The listing builds one solid part. Answer for the finished solid, in the listing's coordinates (mm). Face numbers are marked on the shaded views. Coordinates: 2 decimals unless noted, no trailing zeros. Write each loop counter-clockwise with the first axis right and the second up, starting at its lowest first coordinate (ties: lowest second). Pieces come first, ordered by that corner, then holes.
from build123d import *

# Parameters (mm, degrees)
EXTRUDE_1_DEPTH     = 5
SKETCH_4_R          = 1.5
CUT_EXTRUDE_4_DEPTH = 90.180603272
SKETCH_4_3_W        = 111
SKETCH_4_3_H        = 85
SKETCH_4_3_R        = 1.5
CUT_EXTRUDE_5_DEPTH = 3.3
FILLET_1_R          = 2


with BuildPart() as part:
    # Sketch 2 → Extrude 1 (new body)
    with BuildSketch(Plane(origin=(0, 0, 0), x_dir=(1, 0, 0), z_dir=(0, 1, 0))):
        Polygon((-43.3, 45.3), (-43.3, 67.3), (-33.3, 67.3), (-33.3, 45.3), (33.3, 45.3), (33.3, 67.3), (43.3, 67.3), (43.3, 45.3), (58.3, 45.3), (58.3, -45.3), (-58.3, -45.3), (-58.3, 45.3), align=None)
        with BuildLine():
            Line((-35.55, 62.3), (-35.55, 50.3))
            ThreePointArc((-35.55, 50.3), (-38.3, 47.55), (-41.05, 50.3))
            Line((-41.05, 50.3), (-41.05, 62.3))
            ThreePointArc((-41.05, 62.3), (-38.3, 65.05), (-35.55, 62.3))
        make_face(mode=Mode.SUBTRACT)
        with BuildLine():
            Line((35.55, 62.3), (35.55, 50.3))
            ThreePointArc((35.55, 50.3), (38.3, 47.55), (41.05, 50.3))
            Line((41.05, 50.3), (41.05, 62.3))
            ThreePointArc((41.05, 62.3), (38.3, 65.05), (35.55, 62.3))
        make_face(mode=Mode.SUBTRACT)
    extrude(amount=EXTRUDE_1_DEPTH)

    # Sketch 4 → Cut-Extrude 4 (cut, through all)
    with BuildSketch(Plane(origin=(0, 5, 0), x_dir=(1, 0, 0), z_dir=(0, 1, 0))):
        with Locations(Location((-51.5, 38.5, 0), (0, 0, 270))):
            Circle(SKETCH_4_R)
        with Locations(Location((-51.5, -38.5, 0), (0, 0, 270))):
            Circle(SKETCH_4_R)
        with Locations(Location((51.5, -38.5, 0), (0, 0, 270))):
            Circle(SKETCH_4_R)
        with Locations(Location((51.5, 38.5, 0), (0, 0, 270))):
            Circle(SKETCH_4_R)
    extrude(amount=-CUT_EXTRUDE_4_DEPTH, mode=Mode.SUBTRACT)

    # Sketch 4_3 → Cut-Extrude 5 (cut)
    with BuildSketch(Plane(origin=(0, 5, 0), x_dir=(1, 0, 0), z_dir=(0, 1, 0))):
        Rectangle(SKETCH_4_3_W, SKETCH_4_3_H)
        with Locations(Location((-51.5, -38.5, 0), (0, 0, 270))):
            Circle(SKETCH_4_3_R, mode=Mode.SUBTRACT)
        with Locations(Location((-51.5, 38.5, 0), (0, 0, 270))):
            Circle(SKETCH_4_3_R, mode=Mode.SUBTRACT)
        with Locations(Location((51.5, -38.5, 0), (0, 0, 270))):
            Circle(SKETCH_4_3_R, mode=Mode.SUBTRACT)
        with Locations(Location((51.5, 38.5, 0), (0, 0, 270))):
            Circle(SKETCH_4_3_R, mode=Mode.SUBTRACT)
    extrude(amount=-CUT_EXTRUDE_5_DEPTH, mode=Mode.SUBTRACT)

    # Fillet 1
    fillet_1_edges = [part.edges().sort_by_distance(p)[0] for p in [
        (-58.3, 2.5, -45.3),
        (-43.3, 2.5, -45.3),
        (-43.3, 2.5, -67.3),
        (-33.3, 2.5, -67.3),
        (-33.3, 2.5, -45.3),
        (33.3, 2.5, -45.3),
        (33.3, 2.5, -67.3),
        (43.3, 2.5, -67.3),
        (43.3, 2.5, -45.3),
        (58.3, 2.5, -45.3),
        (58.3, 2.5, 45.3),
        (-58.3, 2.5, 45.3),
    ]]
    fillet(fillet_1_edges, radius=FILLET_1_R)


solid = part.part
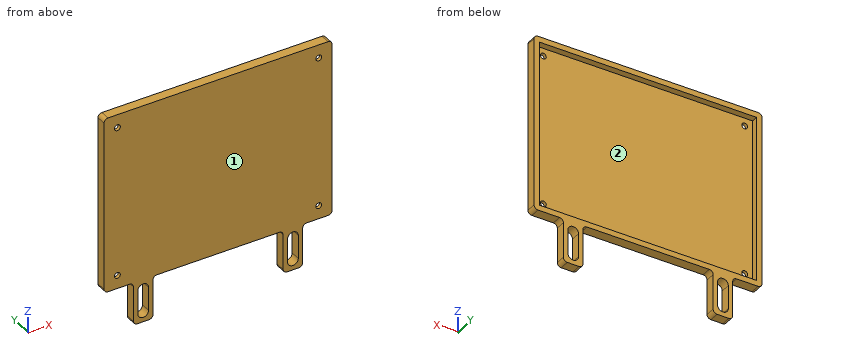
1. Section C-C on x = 38.3 is taken. Give the vertices of the cut face in (y, z).
Results found:
outline: (0, -67.3) - (5, -67.3) - (5, -65.05) - (0, -65.05) - close; (0, -47.55) - (5, -47.55) - (5, -42.5) - (1.7, -42.5) - (1.7, 42.5) - (5, 42.5) - (5, 45.3) - (0, 45.3) - close
2. Section D-D on x = -6 is taken. Give the vertices of the cut face in (y, z).
Results found:
outline: (0, -45.3) - (5, -45.3) - (5, -42.5) - (1.7, -42.5) - (1.7, 42.5) - (5, 42.5) - (5, 45.3) - (0, 45.3) - close
3. Flat-ended cylindrical pins translate along their axes: P1, Ø2.5, axis at x = -10, y = 3, coming from the -Z side; P2, Ø1.5, axis at y = 3, z = -55.5, coming from the -X side; P3, Ø2.5, axis at y = 3.5, z = -54.5, coming from the +X side; P4, Ø2.5, axis at x = 51.5, z = 38.5, coming from the -Y side. Find the tip coordinate at first contact, or state that the pin passes through.
Results found:
P1: stops at z = -45.3
P2: stops at x = -43.3
P3: stops at x = 43.3
P4: passes through
4. Section A-A on z = 38.5 is taken. Give the vertices of the cut face in (x, y), then the cut area to 4 significant figures.
Results found:
outline: (-58.3, 0) - (-53, 0) - (-53, 1.7) - (-55.5, 1.7) - (-55.5, 5) - (-58.3, 5) - close; (-50, 0) - (50, 0) - (50, 1.7) - (-50, 1.7) - close; (53, 0) - (58.3, 0) - (58.3, 5) - (55.5, 5) - (55.5, 1.7) - (53, 1.7) - close
area: 206.5 mm2
5. Section B-B on z = -59.5 is taken. Give the vertices of the cut face in (x, y).
Results found:
outline: (-43.3, 0) - (-41.05, 0) - (-41.05, 5) - (-43.3, 5) - close; (-35.55, 0) - (-33.3, 0) - (-33.3, 5) - (-35.55, 5) - close; (33.3, 0) - (35.55, 0) - (35.55, 5) - (33.3, 5) - close; (41.05, 0) - (43.3, 0) - (43.3, 5) - (41.05, 5) - close
6. For a pull along X with two mould halves and no side action, classify the marked faces 1 and 2 as pulls with the +X half, pulls with the -X half, needs draft (parallel to the pull), parting line crosses it, or undercut.
Results found:
face 1: needs draft
face 2: undercut
7. Find the intervals of material crossed by L1, parallel to X at y = 0.8, z = -54; L2, parallel to Z at x = -46, y = 3.3; L3, parallel to X at y = 2.65, z = -42, in increasing order.
Results found:
L1: x = -43.3 to -41.05, -35.55 to -33.3, 33.3 to 35.55, 41.05 to 43.3
L2: z = -45.3 to -42.5, 42.5 to 45.3
L3: x = -58.3 to -55.5, 55.5 to 58.3
